```python
from build123d import *

# Parameters (mm, degrees)
SKETCH1_R           = 15
BOSS_EXTRUDE1_DEPTH = 5
SKETCH2_R           = 1.25
CUT_EXTRUDE1_DEPTH  = 6
SKETCH3_R           = 6
BOSS_EXTRUDE2_DEPTH = 1.5
SKETCH4_R           = 1.5
CUT_EXTRUDE2_DEPTH  = 1.5
CHAMFER5_SIZE       = 0.25
SKETCH5_R           = 4
CUT_EXTRUDE3_DEPTH  = 6
CHAMFER7_SIZE       = 0.5


with BuildPart() as part:
    # Sketch1 → Boss-Extrude1 (new body)
    with BuildSketch(Plane(origin=(0, 0, 0), x_dir=(1, 0, 0), z_dir=(0, 1, 0))):
        Circle(SKETCH1_R)
    extrude(amount=BOSS_EXTRUDE1_DEPTH)

    # Sketch2 → Cut-Extrude1 (cut, through all)
    with BuildSketch(Plane(origin=(0, 5, 0), x_dir=(1, 0, 0), z_dir=(0, 1, 0))):
        with Locations((0, 12)):
            Circle(SKETCH2_R)
        with Locations((-12, 0)):
            Circle(SKETCH2_R)
        with Locations((0, -12)):
            Circle(SKETCH2_R)
        with Locations((12, 0)):
            Circle(SKETCH2_R)
        with Locations((-8.5, 8.5)):
            Circle(SKETCH2_R)
        with Locations((-8.5, -8.5)):
            Circle(SKETCH2_R)
        with Locations((8.5, 8.5)):
            Circle(SKETCH2_R)
        with Locations((8.5, -8.5)):
            Circle(SKETCH2_R)
    extrude(amount=-CUT_EXTRUDE1_DEPTH, mode=Mode.SUBTRACT)

    # Sketch3 → Boss-Extrude2 (add)
    with BuildSketch(Plane(origin=(0, 0, 0), x_dir=(1, 0, 0), z_dir=(0, 1, 0))):
        Circle(SKETCH3_R)
    extrude(amount=-BOSS_EXTRUDE2_DEPTH)

    # Sketch4 → Cut-Extrude2 (cut)
    with BuildSketch(Plane.XZ.offset(1.5)):
        Circle(SKETCH4_R)
    extrude(amount=-CUT_EXTRUDE2_DEPTH, mode=Mode.SUBTRACT)

    # Chamfer5
    chamfer5_edges = [part.edges().sort_by_distance(p)[0] for p in [
        (-1.25, 0, -12),
        (-1.25, 5, -12),
        (7.25, 0, 8.5),
        (7.25, 5, 8.5),
        (7.25, 0, -8.5),
        (7.25, 5, -8.5),
        (-9.75, 0, -8.5),
        (-9.75, 5, -8.5),
        (-13.25, 0, 0),
        (-13.25, 5, 0),
        (-1.25, 0, 12),
        (-1.25, 5, 12),
        (10.75, 0, 0),
        (10.75, 5, 0),
        (-9.75, 0, 8.5),
        (-9.75, 5, 8.5),
    ]]
    chamfer(chamfer5_edges, length=CHAMFER5_SIZE)

    # Sketch5 → Cut-Extrude3 (cut)
    with BuildSketch(Plane(origin=(0, 5, 0), x_dir=(1, 0, 0), z_dir=(0, 1, 0))):
        Circle(SKETCH5_R)
    extrude(amount=-CUT_EXTRUDE3_DEPTH, mode=Mode.SUBTRACT)

    # Chamfer7
    chamfer7_edges = [part.edges().sort_by_distance(p)[0] for p in [
        (-4, 5, 0),
    ]]
    chamfer(chamfer7_edges, length=CHAMFER7_SIZE)


solid = part.part
```
Input: part model. Units: mm. Frame: model coordinates. A direction names the side the tool comes from. Give positions to 0.01 mm unless a question says otherwise; leave off trailing zeros. Write each loop counter-clockwise with the first axis right and the second up, starting at its lowest first coordinate (ties: lowest second). Pieces come first, ordered by that corner, then holes. Notation, with made-up numbers: (50.25, -21.75) - (76.25, -21.75) arc R22 ccw to (76.25, -8.75) - close; hole circle Ø1 at (53, 16.25). An arc over 180 degrees is marked (long way). Write item = value, one per line. Start each with the question number.
1. Section query C-C, the plane z = 0. Count the separate pieces of the cut face and the enclosed holes in it, then the cut area to 3 significant figures.
2. Access query for faces 1 (the cylindrical face through (-0.867, 1.788, 3.905)), 2 (the cylindrical face through (-9.49, 2.53, 9.26)). Directions: +Z, -Z, +X, -X, +Y, -Y. A direction counts if a zero-diameter tool reaches every point of the face in a straight line with its end or side. Return the directions, or none.
3. Section query B-B, the plane x = -12. Output: boundary loops of the cut face in (y, z), then the cut area to 3 significant figures.
4. Mould query, pull axis X, two halves, no side actions, for faces 3 (the cylindrical face through (-0.16, 2.53, 10.76)), 4 (the flat face through (3, 5, -4)). Classes: released by +X, released by -X, zero draft, split by the parting line, or undercut.
5. Ray query, L1, parallel to Z at x = 0, y = 2.1; L2, parallel to X at y = 0.5, z = 8.5; L3, parallel to X at y = -0.5, z = 0.75. Return the intervals inside material, ascending.
6. First-contact query: pin 1 Ø2 at (x, z) = (0, -12) entering from -Y; pin 2 Ø4 at (x, z) = (8.5, 8.5) entering from -Y; pin 3 Ø3 at (y, z) = (3, 10.5) entering from -X; pin 4 Ø3 at (x, y) = (6, 0.5) entering from +Z. Flat tips, straight axial feed; report the tip coordinate or a pass-through.
7. Section query A-A, the plane z = 12. Output: boundary loops of the cut face in (x, y), then the cut area to 3 significant figures.
Check sheet entries:
q1.separate_pieces = 4
q1.enclosed_holes = 0
q1.area = 93.0 mm2
q2.face_1 = +Y
q2.face_2 = +Y, -Y
q3.outline = (0, -9) - (5, -9) - (5, -1.5) - (4.75, -1.25) - (0.25, -1.25) - (0, -1.5) - close; (0, 1.5) - (0.25, 1.25) - (4.75, 1.25) - (5, 1.5) - (5, 9) - (0, 9) - close
q3.area = 77.4 mm2
q4.face_3 = undercut
q4.face_4 = zero draft
q5.L1 = -15 to -13.25, -10.75 to -4, 4 to 10.75, 13.25 to 15
q5.L2 = -12.36 to -9.75, -7.25 to 7.25, 9.75 to 12.36
q5.L3 = -5.95 to -3.93, 3.93 to 5.95
q6.pin_1 = through
q6.pin_2 = 0
q6.pin_3 = -12
q6.pin_4 = 14.31
q7.outline = (-9, 0) - (-1.5, 0) - (-1.25, 0.25) - (-1.25, 4.75) - (-1.5, 5) - (-9, 5) - close; (1.25, 0.25) - (1.5, 0) - (9, 0) - (9, 5) - (1.5, 5) - (1.25, 4.75) - close
q7.area = 77.4 mm2
